from build123d import *

# Parameters (mm, degrees)
SKETCH1_R           = 19
BOSS_EXTRUDE1_DEPTH = 36
SKETCH2_R           = 18.75
BOSS_EXTRUDE2_DEPTH = 36
SKETCH3_R           = 19
BOSS_EXTRUDE3_DEPTH = 56
SKETCH4_R           = 37.5
BOSS_EXTRUDE4_DEPTH = 51
SKETCH5_R           = 18.25
CUT_EXTRUDE1_DEPTH  = 139.551434493
SKETCH6_W           = 5
SKETCH6_H           = 18.5
SKETCH6_H_2         = 5
SKETCH7_R           = 2.5
CUT_EXTRUDE2_DEPTH  = 9
SKETCH8_R           = 23
CUT_EXTRUDE3_DEPTH  = 4


with BuildPart() as part:
    # Sketch1 → Boss-Extrude1 (new body)
    with BuildSketch(Plane(origin=(0, 0, 0), x_dir=(0, 0, -1), z_dir=(1, 0, 0))):
        Circle(SKETCH1_R)
    extrude(amount=BOSS_EXTRUDE1_DEPTH)

    # Sketch2 → Boss-Extrude2 (add)
    with BuildSketch(Plane(origin=(36, 0, 0), x_dir=(0, 0, -1), z_dir=(1, 0, 0))):
        Circle(SKETCH2_R)
    extrude(amount=BOSS_EXTRUDE2_DEPTH)

    # Sketch3 → Boss-Extrude3 (add)
    with BuildSketch(Plane(origin=(72, 0, 0), x_dir=(0, 0, -1), z_dir=(1, 0, 0))):
        Circle(SKETCH3_R)
    extrude(amount=BOSS_EXTRUDE3_DEPTH)

    # Sketch4 → Boss-Extrude4 (add)
    with BuildSketch(Plane(origin=(128, 0, 0), x_dir=(0, 0, -1), z_dir=(1, 0, 0))):
        Circle(SKETCH4_R)
    extrude(amount=-BOSS_EXTRUDE4_DEPTH)

    # Sketch5 → Cut-Extrude1 (cut, through all)
    with BuildSketch(Plane(origin=(128, 0, 0), x_dir=(0, 0, -1), z_dir=(1, 0, 0))):
        Circle(SKETCH5_R)
    extrude(amount=-CUT_EXTRUDE1_DEPTH, mode=Mode.SUBTRACT)

    # Sketch6 → Cut-Revolve1 (revolve, cut)
    with BuildSketch(Plane.XY, mode=Mode.PRIVATE) as cut_revolve1_sk:
        with Locations((81.5, 28.25)):
            Rectangle(SKETCH6_W, SKETCH6_H)
        with Locations((88.622995217, 28.25)):
            Rectangle(SKETCH6_W, SKETCH6_H)
        with Locations((95.745990433, 28.25)):
            Rectangle(SKETCH6_W, SKETCH6_H)
        with Locations((102.86898565, 28.25)):
            Rectangle(SKETCH6_W, SKETCH6_H)
        with Locations((109.991980867, 28.25)):
            Rectangle(SKETCH6_W, SKETCH6_H)
        with Locations((117.114976083, 28.25)):
            Rectangle(SKETCH6_W, SKETCH6_H)
        with Locations((124.114976083, 35)):
            Rectangle(SKETCH6_W, SKETCH6_H_2)
    revolve(cut_revolve1_sk.sketch.rotate(Axis((0, 0, 0), (1, 0, 0)), 90), axis=Axis((0, 0, 0), (1, 0, 0)), mode=Mode.SUBTRACT)

    # Sketch7 → Cut-Extrude2 (cut)
    with BuildSketch(Plane(origin=(128, 0, 0), x_dir=(0, 0, -1), z_dir=(1, 0, 0))):
        with Locations((0, 27.5)):
            Circle(SKETCH7_R)
        with Locations((27.5, 0)):
            Circle(SKETCH7_R)
        with Locations((0, -27.5)):
            Circle(SKETCH7_R)
        with Locations((-27.5, 0)):
            Circle(SKETCH7_R)
    extrude(amount=-CUT_EXTRUDE2_DEPTH, mode=Mode.SUBTRACT)

    # Sketch8 → Cut-Extrude3 (cut)
    with BuildSketch(Plane(origin=(128, 0, 0), x_dir=(0, 0, -1), z_dir=(1, 0, 0))):
        Circle(SKETCH8_R)
    extrude(amount=-CUT_EXTRUDE3_DEPTH, mode=Mode.SUBTRACT)


solid = part.part
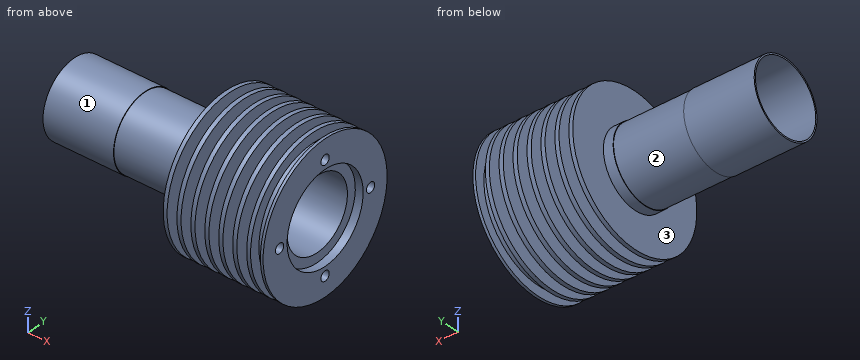
Design review of the part built by this model. Coordinates are the model's own, in mm. Face numbers are marked on the shaded views. Give positions to 0.01 mm unless a question says otherwise; leave off trailing zeros. Write each loop counter-clockwise with the first axis right and the second up, starting at its lowest first coordinate (ties: lowest second). Pieces come first, ordered by that corner, then holes. Notation, with made-up numbers: M 59,58 L 108,58 A22 ccw 108,78 Z; hole C 54.25,-23 d9. An arc over 180 degrees is marked long. Return JSON: item names as keys, results as strings. Group by question number.
Item 1: The part is to be moulded in two halves that separate along X. For the marked faces 1, 2 and 3, say which applies: pulls with the +X half, pulls with the -X half, needs draft (parallel to the pull), parting line crosses it, or undercut.
Item 2: Wall thickness on line 1 along Y through (x, z) = (126.55, 0); line 2 along Y through (x, z) = (122.5, -27.5); line 3 along Z through (x, y) = (63, -1): over which ranges is each line inside the solid? List them lowest first.
Item 3: Take a section at B-B (x = 45.5). Give the boundary of the cut face in (y, z).
Item 4: Clearance check with flat-ended pins moving along their axes: pin 1 Ø5 at (x, y) = (74, 1) entering from -Z; pin 2 Ø3 at (y, z) = (27.5, 0) entering from -X; pin 3 Ø3 at (x, y) = (81.5, -27.5) entering from +Z; pin 4 Ø1.5 at (x, y) = (16.5, 11) entering from -Z. State where each tip first meets the part, or that it passes through.
Item 5: Take a section at A-A (z = 0). Count the separate pieces of the cut face and the enclosed holes in it, plus the area to 3 significant figures.
Return value:
{
 "1": {"face 1": "needs draft", "face 2": "undercut", "face 3": "pulls with the -X half"},
 "2": {"line 1": "y = -32.5 to -30, -25 to -23, 23 to 25, 30 to 32.5", "line 2": "y = -17.32 to -2.5, 2.5 to 17.32", "line 3": "z = -18.72 to -18.22, 18.22 to 18.72"},
 "3": {"outline": "C 0,0 d37.5; hole C 0,0 d36.5"},
 "4": {"pin 1": "stops at z = -19", "pin 2": "stops at x = 77", "pin 3": "passes through", "pin 4": "stops at z = -16"},
 "5": {"separate pieces": "4", "enclosed holes": "0", "area": "779 mm2"}
}
